Part print with two shaded views. Sizes in mm from the minimum x, y, z corner. A direction names the side the tool comes from. Give positions to 0.01 mm unless a question says otherwise; leave off trailing zeros. Write each loop counter-clockwise with the first axis right and the second up, starting at its lowest first coordinate (ties: lowest second). Pieces come first, ordered by that corner, then holes. Notation, with made-up numbers: M -16.5,21 L 25.5,21 A7 ccw 25.5,26 Z; hole C -38,-3 d4. An arc over 180 degrees is marked long. Return JSON: item names as keys, results as strings. Group by question number.
Q1. Band-saw the part on D-D, the plane z = 16.5. Give the cut face in (x, y), then the cut area to 3 significant figures.
Q2. Band-saw the part on B-B, the plane z = 92.5. Give the cut face in (x, y).
Q3. Tool access for the marked faces 1 and 2: list every direction of +Z, -Z, +X, -X, +Y, -Y with a clear straight run to the whole face (end or side of a thin tool).
Q4. Band-saw the part on A-A, the plane x = 116. Give the cut face in (y, z).
Q5. Wall check: probe 1 along X at (y, z) = (0.5, 29.5); probe 2 along X at (y, z) = (0.65, 92.5); probe 3 along Z at (x, y) = (128, 0.6). Give the ranges that are in metal, low to high.
Q6. Pull direction Z, two halves, no side cores. Call the marked faces 3, 4 and 5: +Z half, -Z half, draft (parallel to the pull), parting line (faces both ways), or undercut.
Q7. Band-saw the part on C-C, the plane y = 6.5. Give the cut face in (x, z).
Q8. Flat gauge pins, fed straight in: pin 1 Ø5 at (y, z) = (5, 15.5) entering from +X; pin 2 Ø3.5 at (x, z) = (86, 2.5) entering from -Y; pin 3 Ø7 at (y, z) = (10.5, 7.5) entering from -X; pin 4 Ø2.5 at (x, z) = (7, 29.5) entering from +Y. Where does each tip first touch, or does it go through?
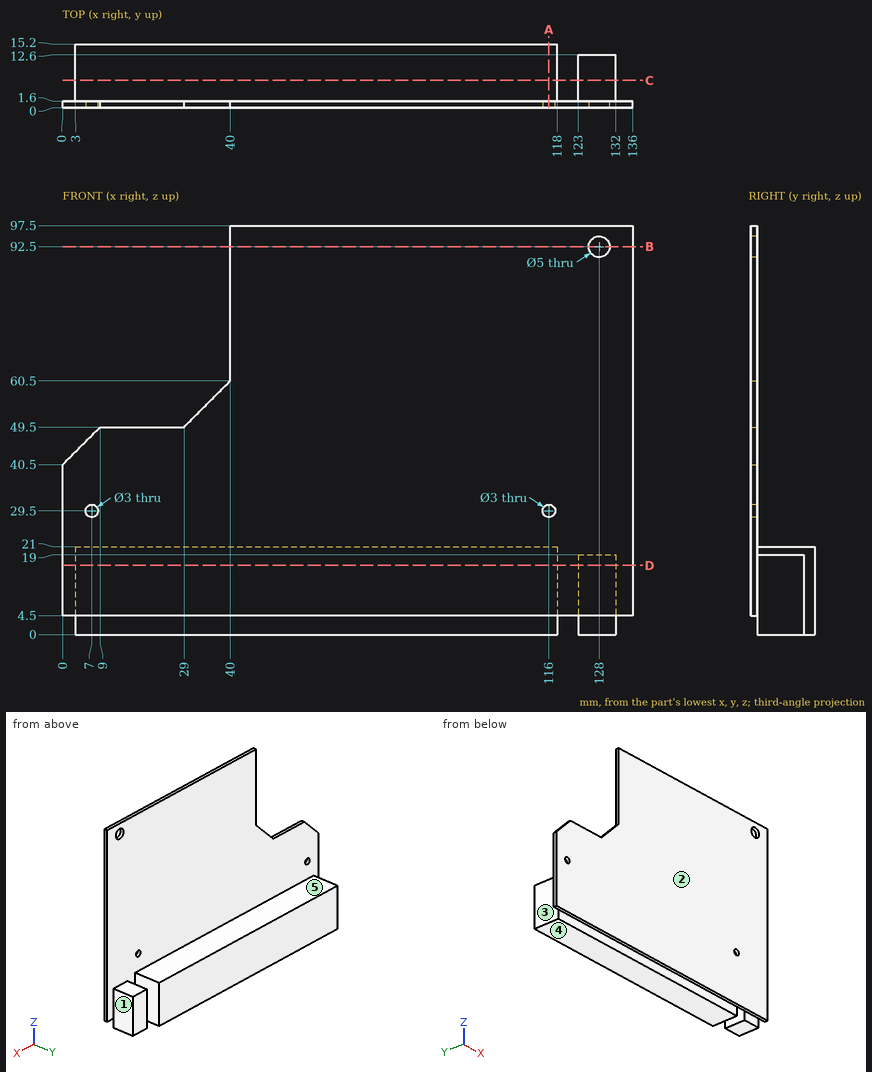
From the geometry:
{
 "1": {"outline": "M 0,0 L 136,0 L 136,1.6 L 132,1.6 L 132,12.6 L 123,12.6 L 123,1.6 L 118,1.6 L 118,15.2 L 3,15.2 L 3,1.6 L 0,1.6 Z", "area": "1,880 mm^2"},
 "2": {"outline": "M 40,0 L 125.5,0 L 125.5,1.6 L 40,1.6 Z; M 130.5,0 L 136,0 L 136,1.6 L 130.5,1.6 Z"},
 "3": {"face 1": "+Z, -Z, +X, +Y", "face 2": "+Z, -Z, +X, -X, -Y"},
 "4": {"outline": "M 0,4.5 L 1.6,4.5 L 1.6,0 L 15.2,0 L 15.2,21 L 1.6,21 L 1.6,28 L 0,28 Z; M 0,31 L 1.6,31 L 1.6,97.5 L 0,97.5 Z"},
 "5": {"probe 1": "x = 0 to 5.5, 8.5 to 114.5, 117.5 to 136", "probe 2": "x = 40 to 125.5, 130.5 to 136", "probe 3": "z = 4.5 to 90, 95 to 97.5"},
 "6": {"face 3": "draft", "face 4": "-Z half", "face 5": "+Z half"},
 "7": {"outline": "M 3,0 L 118,0 L 118,21 L 3,21 Z; M 123,0 L 132,0 L 132,19 L 123,19 Z"},
 "8": {"pin 1": "stops at x = 132", "pin 2": "stops at y = 1.6", "pin 3": "stops at x = 3", "pin 4": "passes through"}
}
